from build123d import *

# Parameters (mm, degrees)
F0_W     = 160
F0_H     = 160
F0_W_2   = 80
F0_H_2   = 25
F0_R     = 40
F1_DEPTH = 19
F0_R_2   = 25
F2_DEPTH = 14
F3_DEPTH = 10


with BuildPart() as f1:
    # F0 (on Top) → F1 (new body)
    with BuildSketch(Plane.XY):
        with Locations((80, 80)):
            Rectangle(F0_W, F0_H)
        with Locations((80, 32.5)):
            Rectangle(F0_W_2, F0_H_2, mode=Mode.SUBTRACT)
        with Locations((80, 100)):
            Circle(F0_R, mode=Mode.SUBTRACT)
    extrude(amount=F1_DEPTH)

    # F0 (on Top) → F2 (join)
    with BuildSketch(Plane.XY):
        with Locations((80, 100)):
            Circle(F0_R)
        with Locations((80, 100)):
            Circle(F0_R_2, mode=Mode.SUBTRACT)
    extrude(amount=F2_DEPTH)

    # F0 (on Top) → F3 (join)
    with BuildSketch(Plane.XY):
        with Locations((80, 32.5)):
            Rectangle(F0_W_2, F0_H_2)
    extrude(amount=F3_DEPTH)


solid = f1.part
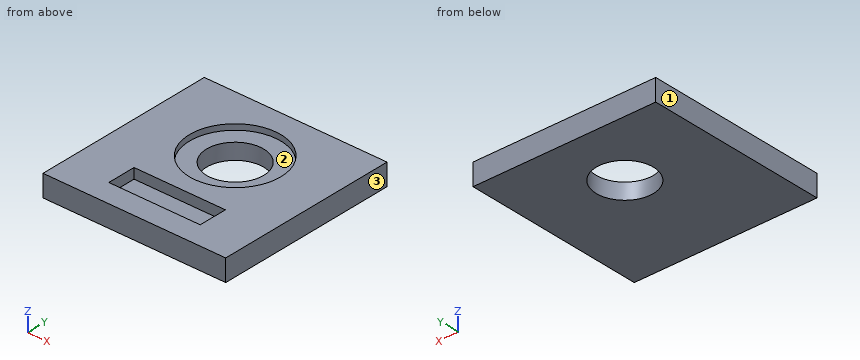
Input: part model. Units: mm. Frame: model coordinates. Face numbers are marked on the shaded views. Give positions to 0.01 mm unless a question says otherwise; leave off trailing zeros. Loops run counter-clockwise (first coordinate to the right, second up) from the corner with the lowest first, then second, coordinate; pieces in that order, holes last. Notation, with made-up numbers: (1, -18.5) - (46, -18.5) arc R28 cw to (46, 18.5) - close; hole circle Ø2 at (-34, -34). An arc over 180 degrees is marked (long way). Use CSV: the item, a comma, the result in double quotes. Start each with the question number.
Item 1: Line query: line 1 (Y direction, x = 80, z = 17.8); line 2 (X direction, y = 35, z = 13); line 3 (Y direction, x = 114.5, z = 12.75). Output: solid intervals per line, ascending.
Item 2: Section D-D on y = 70. Return loops of the section in (x, z), then the cut area to 3 significant figures.
Item 3: Contact query for flat-ended pins moving along their axis: P1, Ø12, axis at x = 129, y = 94, coming from the -Z side; P2, Ø12.5, axis at x = 95.5, y = 38, coming from the +Z side; P3, Ø24, axis at x = 97.5, y = 98, coming from the +Z side. Output: stop coordinate, or through.
Item 4: Section A-A on x = 80. Return loops of the section in (y, z).
Item 5: Section B-B on y = 100. Return loops of the section in (x, z).
Item 6: Mould query, pull axis X, two halves, no side actions, for the marked faces 1, 2 and 3. Classes: pulls with the +X half, pulls with the -X half, needs draft (parallel to the pull), parting line crosses it, or undercut.
Item 7: Section C-C on z = 16.25. Return loops of the section in (x, y), then the cut area to 3 significant figures.
Ans:
1,line 1,"y = 0 to 20, 45 to 60, 140 to 160"
1,line 2,"x = 0 to 40, 120 to 160"
1,line 3,"y = 0 to 20, 45 to 160"
2,outline,"(0, 0) - (160, 0) - (160, 19) - (106.46, 19) - (106.46, 14) - (53.54, 14) - (53.54, 19) - (0, 19) - close"
2,area,"2,780 mm2"
3,P1,"stops at z = 0"
3,P2,"stops at z = 10"
3,P3,"stops at z = 14"
4,outline,"(0, 0) - (75, 0) - (75, 14) - (60, 14) - (60, 19) - (45, 19) - (45, 10) - (20, 10) - (20, 19) - (0, 19) - close; (125, 0) - (160, 0) - (160, 19) - (140, 19) - (140, 14) - (125, 14) - close"
5,outline,"(0, 0) - (55, 0) - (55, 14) - (40, 14) - (40, 19) - (0, 19) - close; (105, 0) - (160, 0) - (160, 19) - (120, 19) - (120, 14) - (105, 14) - close"
6,face 1,"pulls with the -X half"
6,face 2,"undercut"
6,face 3,"pulls with the +X half"
7,outline,"(0, 0) - (160, 0) - (160, 160) - (0, 160) - close; hole (40, 20) - (120, 20) - (120, 45) - (40, 45) - close; hole circle Ø80 at (80, 100)"
7,area,"18,600 mm2"
